Can you work these out from the model? Positions are in its coordinate system, mm. Face numbers are marked on the shaded views. A direction names the side the tool comes from. Coordinates: 2 decimals unless noted, no trailing zeros. Order: outer loops, then holes, each group sorted by start corner. A loop starts at its lowest first (then second) coordinate and runs counter-clockwise, first axis right, second up. Notation, with made-up numbers: (14, 72) - (37, 72) arc R22 ccw to (37, 111) - close; hole circle Ø11 at (-1, 76.5). An arc over 180 degrees is marked (long way). Use a Markdown table: item, result. Add a question column.
(1) On a 3-axis mill with a long thin cutter (end or side, diameter ignored), from which of +Z, -Z, +X, -X, +Y, -Y can I reach the whole of each face in a straight line? I mean the marked faces 1, 2, 3, 4 and 5. Say none if no direction works.
(2) If I drill on L1, parallel to Y at x = -47, z = -18; L2, parallel to X at y = 68.5, z = -24; L3, parallel to Z at x = -8.5, y = 81.5, over which ranges is the centre line in solid material (lowest first)? Write a range as [from, to].
(3) We'd pull the mould along X, two halves only. Please class the marked faces 6, 7 and 8: pulls with the +X half, pulls with the -X half, needs draft (parallel to the pull), parting line crosses it, or undercut.
(4) For pin 1 Ø10 at (x, z) = (-45.5, -26) entering from -Y; pin 2 Ø10 at (x, z) = (-15.5, -14.5) entering from -Y; pin 3 Ø8 at (y, z) = (56.5, -34.5) entering from -X, each with a flat end and sliding along its axis, tell me the tip position at first contact or that it passes through.
(5) I want a section at A-A (y = 58). List the corners of the cut face in (x, z) for me, and give its area (3 significant figures).
(6) I want a section at B-B (y = 75.5). List the corners of the cut face in (x, z) for me.
```python
from build123d import *

# Parameters (mm, degrees)
REVOLUCI_N1_ANGLE       = 90
REVOLUCI_N2_ANGLE       = 20
REVOLUCI_N3_ANGLE       = 20
CORTAR_EXTRUIR1_DEPTH   = 129.015444104
CROQUIS13_R             = 4.5
SALIENTE_EXTRUIR1_DEPTH = 10


with BuildPart() as part:
    # Croquis2 → Revolución1 (revolve)
    with BuildSketch(Plane(origin=(0, 0, 0), x_dir=(0, 0, -1), z_dir=(1, 0, 0))):
        with BuildLine():
            Line((0, 0), (0, 6))
            ThreePointArc((0, 6), (16.315231643, 21.503634207), (26, 41.82))
            Line((26, 41.82), (40.517487246, 96))
            Line((40.517487246, 96), (45.806819571, 96))
            Line((45.806819571, 96), (30.935014244, 40.497666919))
            ThreePointArc((30.935014244, 40.497666919), (19.472326357, 17.189666117), (0, 0))
        make_face()
    revolve(axis=Axis((0, 0, 0), (0, 1, 0)), revolution_arc=REVOLUCI_N1_ANGLE)

    # Croquis10 → Revolución2 (revolve)
    with BuildSketch(Plane(origin=(0, 0, 0), x_dir=(0, 1, 0), z_dir=(0.866025403784438, 0, -0.500000000000001))):
        Polygon((81, -41.787581685), (96, -45.806819571), (96, -60.806819571), (81, -56.787581685), align=None)
    revolve(axis=Axis((0, 0, 0), (0, -1, 0)), revolution_arc=REVOLUCI_N2_ANGLE)

    # Croquis11 → Revolución3 (revolve)
    with BuildSketch(Plane(origin=(0, 0, 0), x_dir=(0, 1, 0), z_dir=(0.499999999999998, 1.4337406519976025e-15, -0.8660254037844398))):
        Polygon((96, -45.806819571), (96, -60.806819571), (81, -56.787581685), (81, -41.787581685), align=None)
    revolve(axis=Axis((0, 0, 0), (0, 1, 0)), revolution_arc=REVOLUCI_N3_ANGLE)

    # Croquis12 → Cortar-Extruir1 (cut, through all)
    with BuildSketch(Plane(origin=(0, 96, 0), x_dir=(1, 0, 0), z_dir=(0, 1, 0))):
        with BuildLine():
            Line((-7.954270743, 45.110911055), (-20.197712047, 57.354352358))
            ThreePointArc((-20.197712047, 57.354352358), (-15.430239205, 58.81646899), (-10.558993408, 59.88302735))
            Line((-10.558993408, 59.88302735), (-7.954270743, 45.110911055))
        make_face()
        with BuildLine():
            Line((-45.110911055, 7.954270743), (-57.354352358, 20.197712047))
            ThreePointArc((-57.354352358, 20.197712047), (-58.81646899, 15.430239205), (-59.88302735, 10.558993408))
            Line((-59.88302735, 10.558993408), (-45.110911055, 7.954270743))
        make_face()
    extrude(amount=-CORTAR_EXTRUIR1_DEPTH, mode=Mode.SUBTRACT)

    # Croquis13 → Saliente-Extruir1 (add)
    with BuildSketch(Plane(origin=(18.578320156, 0, -18.578320156), x_dir=(-0.7071067811865489, 0, -0.7071067811865461), z_dir=(0.7071067811865461, 0, -0.7071067811865489))):
        with Locations(Location((45.056780398, 88.5, 0), (0, 0, 180))):
            Circle(CROQUIS13_R)
    saliente_extruir1 = extrude(amount=SALIENTE_EXTRUIR1_DEPTH)

    # Simetría1: Saliente-Extruir1 across plane
    add(saliente_extruir1.mirror(Plane(origin=(0, 0, 0), x_dir=(0.7071067811865488, 1.170644340293136e-15, 0.7071067811865464), z_dir=(0.7071067811865462, 1.1706443402931319e-15, -0.7071067811865488))))


solid = part.part
```
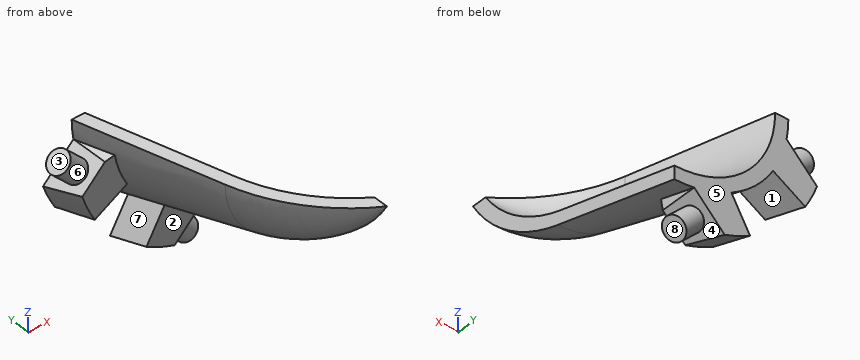
Answers follow:
| question | item | result |
|---|---|---|
| 1 | face 1 | -Z, -Y |
| 1 | face 2 | -Z, -X, -Y |
| 1 | face 3 | +Z, -X, +Y, -Y |
| 1 | face 4 | none |
| 1 | face 5 | +Z, -Z, +X, -X, +Y |
| 2 | L1 | y = [81, 96] |
| 2 | L2 | x = [-30.02, -22.87] |
| 2 | L3 | z = [-45.66, -35.63] |
| 3 | face 6 | undercut |
| 3 | face 7 | pulls with the -X half |
| 3 | face 8 | pulls with the +X half |
| 4 | pin 1 | stops at y = 81 |
| 4 | pin 2 | stops at y = 13.26 |
| 4 | pin 3 | stops at x = -17.94 |
| 5 | outline | (-35.62, 0) arc R35.62 ccw to (0, -35.62) - (0, -30.34) arc R30.34 cw to (-30.34, 0) - close |
| 5 | area | 274 mm² |
| 6 | outline | (-40.31, 0) arc R40.31 ccw to (0, -40.31) - (0, -35.02) arc R35.02 cw to (-35.02, 0) - close |
